Source: three-view drawing plus pictorial views. Frame: mm from the lowest corner of the part. Give positions to 0.01 mm unless a question says otherwise; leave off trailing zeros. Write each loop counter-clockwise with the first axis right and the second up, starting at its lowest first coordinate (ties: lowest second). Pieces come first, ordered by that corner, then holes. Notation, with made-up numbers: M 22,8.25 L 27,8.25 A27 ccw 27,31.25 Z; hole C -28.5,51 d5. An arc over 180 degrees is marked long. Return JSON: item names as keys, results as strings.
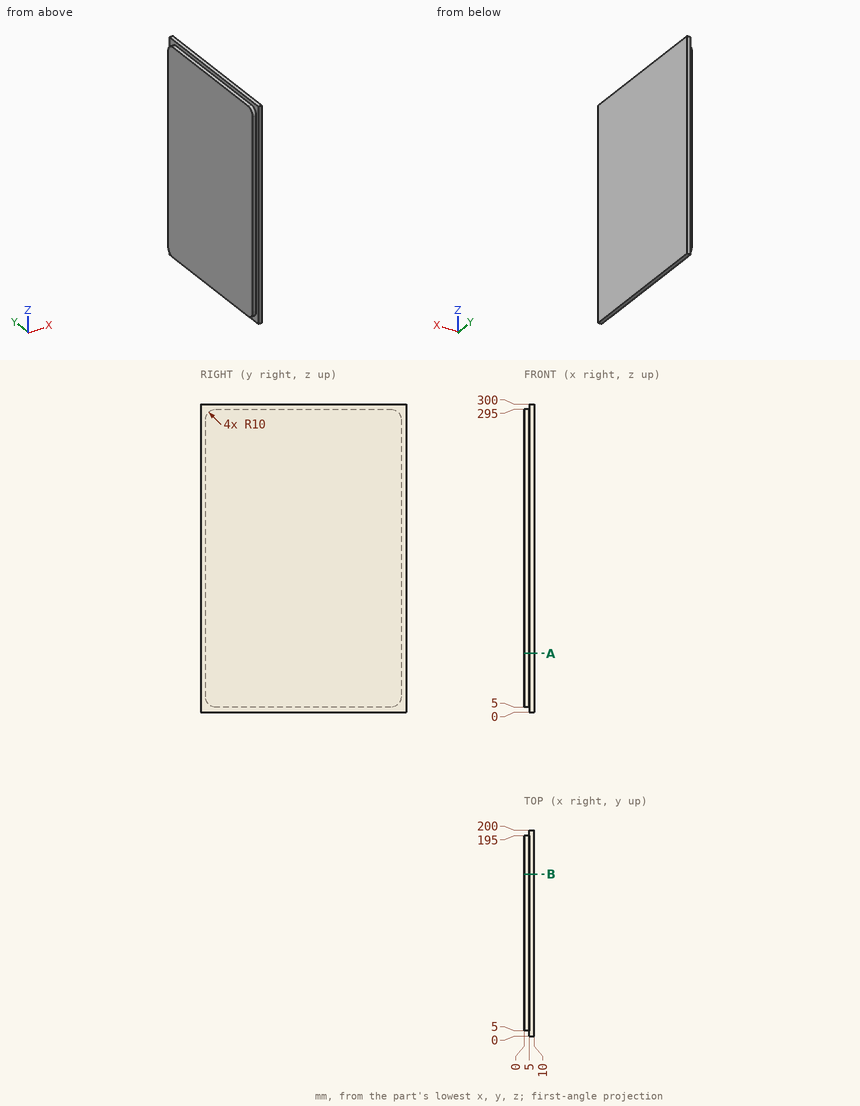
1) Line query: line 1 (Y direction, x = 4, z = 102.5); line 2 (Z direction, x = 4, y = 180.5). Output: solid intervals per line, ascending. Write a range as [from, to].
Numbers:
{"line 1": "y = [5, 195]", "line 2": "z = [5, 295]"}
2) Contact query for flat-ended pins moving along their axis: pin 1 Ø2.5 at (x, y) = (1.5, 121.5) entering from -Z; pin 2 Ø4 at (x, z) = (2, 191) entering from -Y; pin 3 Ø4 at (x, z) = (1.5, 137.5) entering from +Y. Output: stop coordinate, or through.
Numbers:
{"pin 1": "stops at z = 5", "pin 2": "stops at y = 5", "pin 3": "stops at y = 195"}
3) Cut plane B-B, the plane y = 157.5. Return the cut outline in (x, z).
Numbers:
{"outline": "M 0,5 L 5,5 L 5,0 L 10,0 L 10,300 L 5,300 L 5,295 L 0,295 Z"}
4) Cut plane A-A, the plane z = 57.5. Return the cut outline in (x, y), then the cut area to 3 significant figures.
Numbers:
{"outline": "M 0,5 L 5,5 L 5,0 L 10,0 L 10,200 L 5,200 L 5,195 L 0,195 Z", "area": "1,950 mm²"}
